Autodesk Inventor part; units mm, degrees
ref_plane "YZ Plane" through (0, 0, 0) normal (1, 0, 0) x (0, 1, 0)
ref_plane "XZ Plane" through (0, 0, 0) normal (0, 1, 0) x (-1, 0, 0)
ref_plane "XY Plane" through (0, 0, 0) normal (0, 0, 1) x (1, 0, 0)
sketch "Sketch1" plane through (0, 0, 0) normal (0, 0, 1) x (1, 0, 0)
  line L0 (-6.35, -3.6662) -> (-6.35, 3.6662)
  line L1 (-6.35, 3.6662) -> (0, 7.3323)
  line L2 (0, 7.3323) -> (6.35, 3.6662)
  line L3 (6.35, 3.6662) -> (6.35, -3.6662)
  line L4 (6.35, -3.6662) -> (0, -7.3323)
  line L5 (0, -7.3323) -> (-6.35, -3.6662)
  point P0 (0, 0)
  point P1 (0, 0)
  dimension "Size" = 12.7
extrude "Extrusion1" add sketch "Sketch1" along normal mid plane 160.3375
sketch "Sketch3" plane through (0, 0, 80.1688) normal (0, 0, 1) x (1, 0, 0)
  line L0 (-6.35, 3.6662) -> (0, 7.3323) construction
  line L1 (0, 7.3323) -> (6.35, 3.6662) construction
  line L2 (6.35, 3.6662) -> (6.35, -3.6662) construction
  line L3 (6.35, -3.6662) -> (0, -7.3323) construction
  line L4 (0, -7.3323) -> (-6.35, -3.6662) construction
  line L5 (-6.35, -3.6662) -> (-6.35, 3.6662) construction
  point P0 (0, 0)
hole "Hole1" at (0, 0, 80.1688) direction (0, 0, -1) diameter 5.1054 end through all
sketch "Sketch4" plane through (0, 0, 80.1688) normal (0, 0, 1) x (1, 0, 0)
  circle A0 centre (0, 0) radius 2.5527 construction
  line L0 (-6.35, 3.6662) -> (0, 7.3323) construction
  line L1 (0, 7.3323) -> (6.35, 3.6662) construction
  line L2 (6.35, 3.6662) -> (6.35, -3.6662) construction
  line L3 (6.35, -3.6662) -> (0, -7.3323) construction
  line L4 (0, -7.3323) -> (-6.35, -3.6662) construction
  line L5 (-6.35, -3.6662) -> (-6.35, 3.6662) construction
  circle A1 centre (0, 0) radius 6.8771
  circle A2 centre (0, 0) radius 8.89
  dimension "thunder" = 13.7541
  dimension "d16" = 17.78
extrude "Extrusion3" cut sketch "Sketch4" against normal through all
sketch "Sketch5" plane through (0, 0, 80.1688) normal (0, 0, 1) x (1, 0, 0)
  arc A0 (5.4616, -4.1791) -> (6.35, -2.6403) centre (0, 0) ccw
  line L0 (5.4616, -4.1791) -> (0.8884, -6.8194)
  arc A1 (-0.8884, -6.8194) -> (0.8884, -6.8194) centre (0, 0) ccw
  line L1 (-0.8884, -6.8194) -> (-5.4616, -4.1791)
  arc A2 (-6.35, -2.6403) -> (-5.4616, -4.1791) centre (0, 0) ccw
  line L2 (-6.35, -2.6403) -> (-6.35, 2.6403)
  arc A3 (-5.4616, 4.1791) -> (-6.35, 2.6403) centre (0, 0) ccw
  line L3 (-5.4616, 4.1791) -> (-0.8884, 6.8194)
  arc A4 (0.8884, 6.8194) -> (-0.8884, 6.8194) centre (0, 0) ccw
  line L4 (0.8884, 6.8194) -> (5.4616, 4.1791)
  arc A5 (6.35, 2.6403) -> (5.4616, 4.1791) centre (0, 0) ccw
  line L5 (6.35, 2.6403) -> (6.35, -2.6403)
  circle A6 centre (0, 0) radius 2.5527
  circle A7 centre (0, 0) radius 6.35
  point P0 (-3.175, 5.4993)
  point P1 (3.175, 5.4993)
  point P2 (6.35, 0)
  point P3 (-6.35, 0)
  point P4 (-3.175, -5.4993)
  point P5 (3.175, -5.4993)
  dimension "d19" = 12.7
extrude "Extrusion4" cut sketch "Sketch5" against normal blind 8.001 contours L0 A7 L5 A0 | L0 A1 L1 A7 | A7 L4 A5 L5 | L1 A2 L2 A7 | A7 L3 A4 L4 | L2 A3 L3 A7
equation "\"bearing\" = 25.4"
properties part number "CL4-020" material "Aluminum 6061"
Part model, mm, in its own coordinate system. A direction names the side the tool comes from. Round coordinates to 2 decimals unless told otherwise and drop trailing zeros. Loops run counter-clockwise (first coordinate to the right, second up) from the corner with the lowest first, then second, coordinate; pieces in that order, holes last.
Item 1: 3-axis set-ups, long thin cutter, end or side, ignore diameter. For faces 4 (the face through (6, -3, 72.168)), 5 (the face through (-6, 3, 72.168)), 6 (the face through (-6, -3, 72.168)), 7 (the face through (3.21, -5.48, -5.07)), 8 (the face through (-1.38, -6.2, 76.22)): which of +Z, -Z, +X, -X, +Y, -Y reach the whole face in a straight line?
Item 2: Drop flat-ended pins along their axis: P1, Ø3, axis at x = 3.5, z = -24, coming from the -Y side; P2, Ø1.5, axis at x = 4.5, z = -17, coming from the +Y side. Give the stop position or say it passes through.
Item 3: Mould opens along Y. For faces 1 (the face through (-3.21, 5.48, -5.07)), 2 (the face through (-0.767, -2.435, -1.122)), 3 (the face through (6, 3, 72.168)) say: +Y half, -Y half, draft (parallel to the pull), parting line (faces both ways), or undercut.
Item 4: Drill centre lines: line 1 (Y direction, x = 0, z = 2); line 2 (X direction, y = 0.25, z = 45.5); line 3 (X direction, y = 0, z = 38). Where is each one in solid material? Low to high.
Item 5: Cut at A-A, the plane z = -48.5. Give the cut face in (x, y).
A:
1. face 4: +Z, +X, -Y
1. face 5: +Z, -X, +Y
1. face 6: +Z, -X, -Y
1. face 7: +Z, -Z, +X, -Y
1. face 8: +Z
2. P1: stops at y = -6.18
2. P2: stops at y = 5.17
3. face 1: +Y half
3. face 2: undercut
3. face 3: draft
4. line 1: y = -6.88 to -2.55, 2.55 to 6.88
4. line 2: x = -6.35 to -2.54, 2.54 to 6.35
4. line 3: x = -6.35 to -2.55, 2.55 to 6.35
5. outline: (-6.35, -2.64) arc R6.88 ccw to (-5.46, -4.18) - (-0.89, -6.82) arc R6.88 ccw to (0.89, -6.82) - (5.46, -4.18) arc R6.88 ccw to (6.35, -2.64) - (6.35, 2.64) arc R6.88 ccw to (5.46, 4.18) - (0.89, 6.82) arc R6.88 ccw to (-0.89, 6.82) - (-5.46, 4.18) arc R6.88 ccw to (-6.35, 2.64) - close; hole circle Ø5.11 at (0, 0)
